Check sheet for the modelled part. Datum: model origin and axes. Units: mm. Face numbers are marked on the shaded views. A direction names the side the tool comes from. Give positions to 0.01 mm unless a question says otherwise; leave off trailing zeros. Loops run counter-clockwise (first coordinate to the right, second up) from the corner with the lowest first, then second, coordinate; pieces in that order, holes last. Notation, with made-up numbers: M -13,19 L 30,19 A17 ccw 30,52 Z; hole C 34,25 d10. An arc over 180 degrees is marked long. Use one line per item in the form item = value.
from build123d import *

# Parameters (mm, degrees)
SKETCH1_W           = 280
SKETCH1_H           = 755
BOSS_EXTRUDE1_DEPTH = 588
SKETCH4_R           = 81
BOSS_EXTRUDE2_DEPTH = 20
BOSS_EXTRUDE3_START = 20
SKETCH4_3_R         = 65
BOSS_EXTRUDE3_DEPTH = 106
BOSS_EXTRUDE4_START = 126
SKETCH4_4_R         = 37
BOSS_EXTRUDE4_DEPTH = 13
BOSS_EXTRUDE5_DEPTH = 268
BOSS_EXTRUDE6_DEPTH = 178
SKETCH7_W           = 55
SKETCH7_H           = 205
BOSS_EXTRUDE7_DEPTH = 55


with BuildPart() as part:
    # Sketch1 → Boss-Extrude1 (new body)
    with BuildSketch(Plane.XY):
        with Locations((-140, 377.5)):
            Rectangle(SKETCH1_W, SKETCH1_H)
    extrude(amount=BOSS_EXTRUDE1_DEPTH)

    # Sketch4 → Boss-Extrude2 (add)
    with BuildSketch(Plane.XZ):
        with Locations(Location((-160, 425, 0), (0, 0, 90))):
            Circle(SKETCH4_R)
    extrude(amount=BOSS_EXTRUDE2_DEPTH)

    # Sketch4<3> → Boss-Extrude3 (add)
    with BuildSketch(Plane.XZ.offset(BOSS_EXTRUDE3_START)):
        with Locations(Location((-160, 425, 0), (0, 0, 270))):
            Circle(SKETCH4_3_R)
    extrude(amount=BOSS_EXTRUDE3_DEPTH)

    # Sketch4<4> → Boss-Extrude4 (add)
    with BuildSketch(Plane.XZ.offset(BOSS_EXTRUDE4_START)):
        with Locations(Location((-160, 425, 0), (0, 0, 90))):
            Circle(SKETCH4_4_R)
    extrude(amount=BOSS_EXTRUDE4_DEPTH)

    # Sketch5 → Boss-Extrude5 (add)
    with BuildSketch(Plane(origin=(0, 0, 268), x_dir=(-1, 0, 0), z_dir=(0, 0, -1))):
        Polygon((0, 0), (-83, 0), (-227, 240.133296317), (-227, 755), (0, 755), align=None)
    extrude(amount=BOSS_EXTRUDE5_DEPTH)

    # Sketch6 → Boss-Extrude6 (add)
    with BuildSketch(Plane.XY.offset(178)):
        Polygon((-280, 0), (0, 0), (0, -70), (-315, -70), (-315, 755), (-280, 755), align=None)
    extrude(amount=-BOSS_EXTRUDE6_DEPTH)

    # Sketch7 → Boss-Extrude7 (add)
    with BuildSketch(Plane.XZ):
        with Locations((-27.5, 370.5)):
            Rectangle(SKETCH7_W, SKETCH7_H)
    extrude(amount=BOSS_EXTRUDE7_DEPTH)


solid = part.part
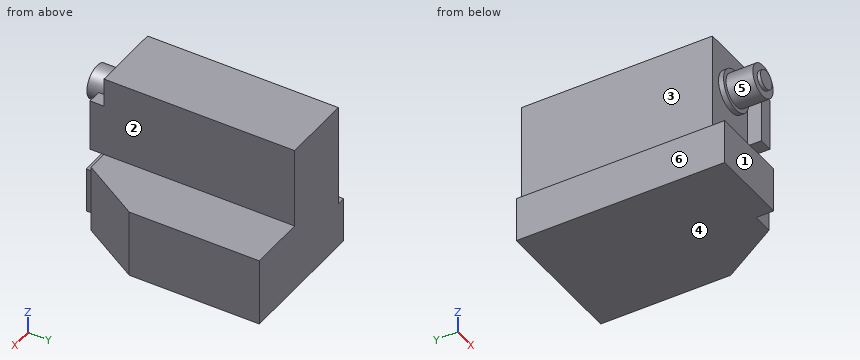
1) Scan lines: line 1 (Z direction, x = 164.5, y = 342); line 2 (X direction, y = 34.5, z = 376.5); line 3 (Y direction, x = -88.5, z = 479.5). Record each from-to range of solid material in increasing order.
Evaluation:
line_1 = 0 to 268
line_2 = -280 to 0
line_3 = 0 to 755
2) Release check for a two-part mould opening along X. For the marked faces 4, 5 and 6 record: pulls with the +X half, pulls with the -X half, needs draft (parallel to the pull), parting line crosses it, or undercut.
Evaluation:
face_4 = needs draft
face_5 = undercut
face_6 = pulls with the -X half
3) Depth check by flat-ended pin: pin 1 Ø8 at (y, z) = (615, 283.5) entering from +X; pin 2 Ø2 at (y, z) = (19, 266) entering from -X; pin 3 Ø5 at (x, y) = (84, 512.5) entering from +Z. Enter the tip coordinate at first touch or a pass-through.
Evaluation:
pin_1 = 0
pin_2 = -280
pin_3 = 268
4) Section check D-D (z = 425). Record the cut outline in (x, y), then the cut area to 3 significant figures.
Evaluation:
outline = M -280,0 L -241,0 L -241,-20 L -225,-20 L -225,-126 L -197,-126 L -197,-139 L -123,-139 L -123,-126 L -95,-126 L -95,-20 L -79,-20 L -79,0 L -55,0 L -55,-55 L 0,-55 L 0,755 L -280,755 Z
area = 232,000 mm^2
5) Section check C-C (z = 83). Record the cut outline in (x, y), then the cut area to 3 significant figures.
Evaluation:
outline = M -315,-70 L 0,-70 L 0,0 L 83,0 L 227,240.13 L 227,755 L -315,755 Z
area = 414,000 mm^2
6) Section check B-B (y = 573.5). Record the cut outline in (x, z), then the cut area to 3 significant figures.
Evaluation:
outline = M -315,0 L 227,0 L 227,268 L 0,268 L 0,588 L -280,588 L -280,178 L -315,178 Z
area = 232,000 mm^2
7) Set-up check for the marked faces 1, 2 and 3: record each of +Z, -Z, +X, -X, +Y, -Y from which the full face is reachable in a straight line by a thin tool's end or side.
Evaluation:
face_1 = -Z, +X, -X, -Y
face_2 = +Z, +X, +Y, -Y
face_3 = +Z, -X, +Y, -Y
8) Section check A-A (x = -160). Record the cut outline in (y, z), then the cut area to 3 significant figures.
Evaluation:
outline = M -139,388 L -126,388 L -126,360 L -20,360 L -20,344 L 0,344 L 0,178 L -70,178 L -70,0 L 755,0 L 755,588 L 0,588 L 0,506 L -20,506 L -20,490 L -126,490 L -126,462 L -139,462 Z
area = 474,000 mm^2
